Geometry: see drawing. Coordinates: mm, zero at the bounding-box minimum. Give positions to 0.01 mm unless a question says otherwise; leave off trailing zeros. Loops run counter-clockwise (first coordinate to the right, second up) from the corner with the lowest first, then second, coordinate; pieces in that order, holes last. Notation, with made-up numbers: (2, 38.5) -> (52, 38.5) arc R14 ccw to (52, 54.5) -> close; hole circle Ø7 at (85.5, 4.5). An arc over 180 degrees is marked (long way). Answer in a Markdown table with one row per item. Add a question column.
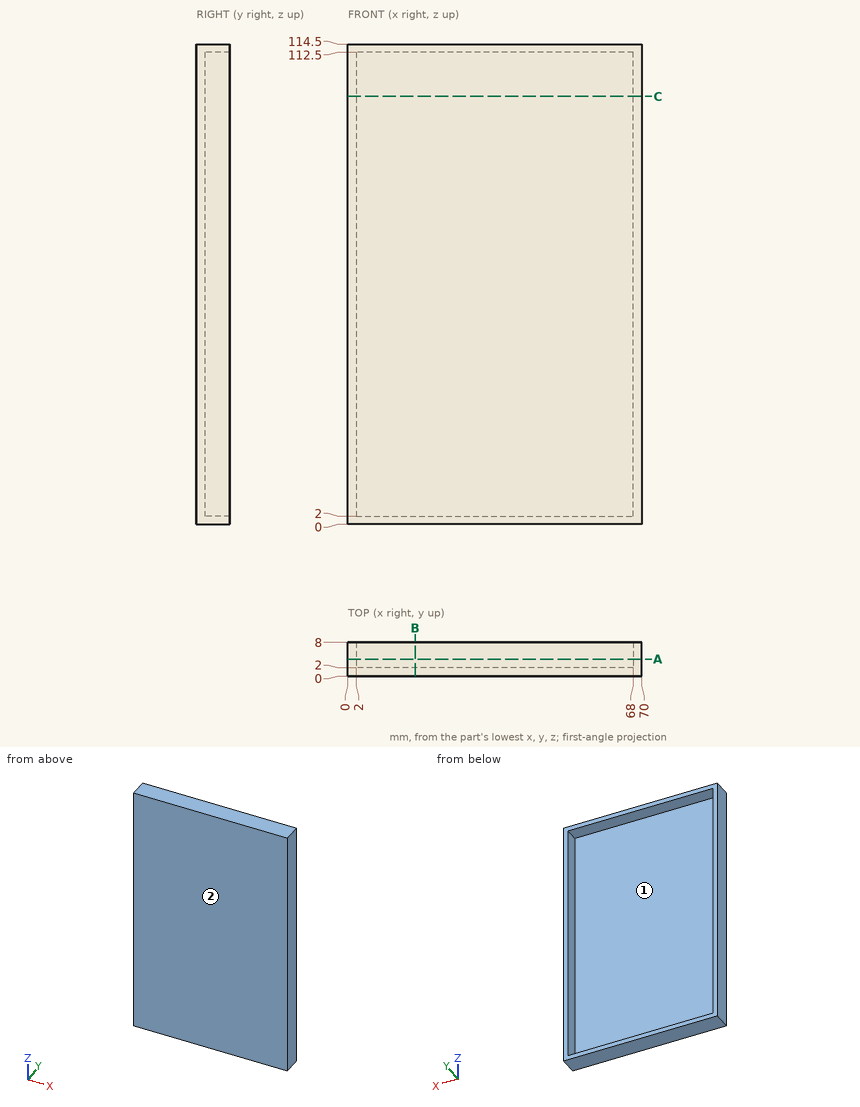
1) Pin query (flat end, axial travel): pin 1 (8 mm diameter, centred on x = 36.5, z = 49.5, fed in from +Y). Return the tip coordinate at first contact, or that it passes through.
2) Section C-C on z = 102. Output: boundary loops of the cut face in (x, y), and give its area (3 significant figures).
3) Section B-B on x = 16. Output: boundary loops of the cut face in (y, z), and give its area (3 significant figures).
4) Section A-A on y = 4. Output: boundary loops of the cut face in (x, z).
5) Pull-direction query (Z, two-part tool) for the marked faces 1 and 2; classes: +Z half, -Z half, draft (parallel to the pull), parting line (faces both ways), or undercut.
6) Material intervals for line 1 along Z through (x, y) = (48.5, 3); line 2 along X through (y, z) = (2.5, 26); line 3 along Y through (x, z) = (46, 23.5), sorted ascending.
Working result:
| question | item | result |
|---|---|---|
| 1 | pin 1 | stops at y = 2 |
| 2 | outline | (0, 0) -> (70, 0) -> (70, 8) -> (68, 8) -> (68, 2) -> (2, 2) -> (2, 8) -> (0, 8) -> close |
| 2 | area | 164 mm2 |
| 3 | outline | (0, 0) -> (8, 0) -> (8, 2) -> (2, 2) -> (2, 112.5) -> (8, 112.5) -> (8, 114.5) -> (0, 114.5) -> close |
| 3 | area | 253 mm2 |
| 4 | outline | (0, 0) -> (70, 0) -> (70, 114.5) -> (0, 114.5) -> close; hole (2, 2) -> (68, 2) -> (68, 112.5) -> (2, 112.5) -> close |
| 5 | face 1 | undercut |
| 5 | face 2 | draft |
| 6 | line 1 | z = 0 to 2, 112.5 to 114.5 |
| 6 | line 2 | x = 0 to 2, 68 to 70 |
| 6 | line 3 | y = 0 to 2 |
